Work out the finished part from the listing and answer in its coordinate system (mm). Coordinates: 2 decimals unless noted, no trailing zeros. Order: outer loops, then holes, each group sorted by start corner. A loop starts at its lowest first (then second) coordinate and runs counter-clockwise, first axis right, second up. Notation, with made-up numbers: M 67,60.5 L 101,60.5 A12 cw 101,72.5 Z; hole C 66,84 d9. An arc over 180 degrees is marked long. Use a Markdown table: item, result. Add a question column.
from build123d import *

# Parameters (mm, degrees)
BOSS_EXTRUDE1_DEPTH = 19.05
CUT_EXTRUDE1_DEPTH  = 20.05


with BuildPart() as part:
    # Sketch1 → Boss-Extrude1 (new body)
    with BuildSketch(Plane.XY):
        Polygon((559.054, 0), (-18.796, 965.516993591), (-18.796, 891.326264322), (514.651764521, 0), align=None)
    extrude(amount=-BOSS_EXTRUDE1_DEPTH)

    # Sketch2 → Cut-Extrude1 (cut, through all)
    with BuildSketch(Plane.XY):
        Polygon((-18.796, 965.516993591), (-18.796, 933.686763034), (0.254, 933.686763034), align=None)
    extrude(amount=-CUT_EXTRUDE1_DEPTH, mode=Mode.SUBTRACT)


solid = part.part
(1) A cutting plane is placed at B-B on y = 75. Write down the section's boundary in (x, z), plus the area to 3 significant figures.
(2) A cutting plane is placed at A-A on z = -13.25. Write down the section's boundary in (x, y), plus the area to 3 significant figures.
(3) A cutting plane is placed at C-C on x = 412. Write down the section's boundary in (y, z).
(4) Given P1, Ø4, axis at y = 577, z = -13.5, coming from the +X side; P2, Ø3, axis at y = 338.5, z = -7, coming from the -X side; P3, Ø3, axis at x = 78, z = -7, coming from the +Y side, each flat-ended and moving along its own axis, determine where each tip first touches the part or whether it passes through.
(5) Straight lines are drawn through the part: line 1 (X direction, y = 811.5, z = -9.75); line 2 (X direction, y = 370.5, z = -9.25); line 3 (Y direction, x = 78.5, z = -3). For each, find the intervals that lie inside material, in ascending order.
From the geometry:
| question | item | result |
|---|---|---|
| 1 | outline | M 469.77,-19.05 L 514.17,-19.05 L 514.17,0 L 469.77,0 Z |
| 1 | area | 846 mm2 |
| 2 | outline | M -18.8,891.33 L 514.65,0 L 559.05,0 L 0.25,933.69 L -18.8,933.69 Z |
| 2 | area | 40,900 mm2 |
| 3 | outline | M 171.52,-19.05 L 245.71,-19.05 L 245.71,0 L 171.52,0 Z |
| 4 | P1 | stops at x = 214.92 |
| 4 | P2 | stops at x = 311.17 |
| 4 | P3 | stops at y = 806.29 |
| 5 | line 1 | x = 28.98 to 73.38 |
| 5 | line 2 | x = 292.91 to 337.31 |
| 5 | line 3 | y = 728.76 to 802.95 |
